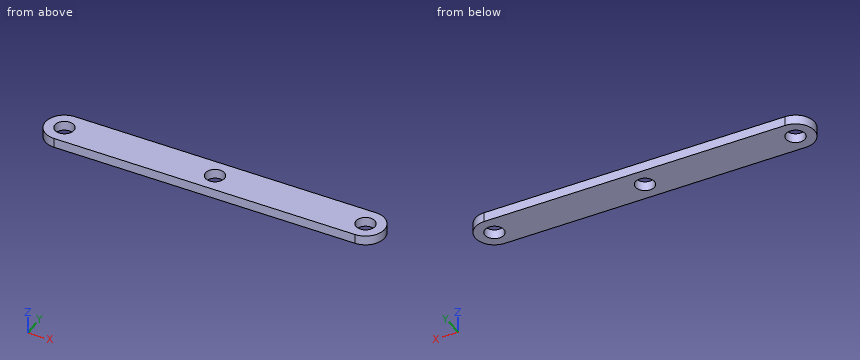
```python
from build123d import *

# Parameters (mm, degrees)
SKETCH1_R           = 3.175
BOSS_EXTRUDE1_DEPTH = 3.175


with BuildPart() as part:
    # Sketch1 → Boss-Extrude1 (new body)
    with BuildSketch(Plane.XY):
        with BuildLine():
            Line((0, 6.35), (101.6, 6.35))
            ThreePointArc((101.6, 6.35), (107.95, 0), (101.6, -6.35))
            Line((101.6, -6.35), (0, -6.35))
            ThreePointArc((0, -6.35), (-6.35, 0), (0, 6.35))
        make_face()
        Circle(SKETCH1_R, mode=Mode.SUBTRACT)
        with Locations((101.6, 0)):
            Circle(SKETCH1_R, mode=Mode.SUBTRACT)
        with Locations((50.8, 0)):
            Circle(SKETCH1_R, mode=Mode.SUBTRACT)
    extrude(amount=BOSS_EXTRUDE1_DEPTH)


solid = part.part
```
Verification items for the finished model (mm, model axes). Give positions to 0.01 mm unless a question says otherwise; leave off trailing zeros. Loops run counter-clockwise (first coordinate to the right, second up) from the corner with the lowest first, then second, coordinate; pieces in that order, holes last. Notation, with made-up numbers: M -9.75,86 L 20.25,86 A13 ccw 20.25,92 Z; hole C -20.75,19 d11. An arc over 180 degrees is marked long. One line per question, with ' | ' between items.
Item 1: Section check A-A, the plane x = 50.8. Record the cut outline in (y, z) (3 decimals), plus the area to 3 significant figures.
Completed:
outline: M -6.35,0 L -3.175,0 L -3.175,3.175 L -6.35,3.175 Z; M 3.175,0 L 6.35,0 L 6.35,3.175 L 3.175,3.175 Z | area: 20.2 mm^2
Item 2: Section check B-B, the plane z = 1.25. Record the cut outline in (x, y) (3 decimals), plus the area to 3 significant figures.
Completed:
outline: M 0,-6.35 L 101.6,-6.35 A6.35 ccw 101.6,6.35 L 0,6.35 A6.35 ccw Z; hole C 0,0 d6.35; hole C 50.8,0 d6.35; hole C 101.6,0 d6.35 | area: 1,320 mm^2
Item 3: Depth check by flat-ended pin: P1, Ø5.5, axis at x = 50.8, y = 0, coming from the -Z side; P2, Ø1, axis at y = -4.5, z = 2, coming from the +X side. Enter the tip coordinate at first touch or a pass-through.
Completed:
P1: passes through | P2: stops at x = 106.53
Item 4: Section check C-C, the plane y = 0. Record the cut outline in (x, z) (3 decimals).
Completed:
outline: M -6.35,0 L -3.175,0 L -3.175,3.175 L -6.35,3.175 Z; M 3.175,0 L 47.625,0 L 47.625,3.175 L 3.175,3.175 Z; M 53.975,0 L 98.425,0 L 98.425,3.175 L 53.975,3.175 Z; M 104.775,0 L 107.95,0 L 107.95,3.175 L 104.775,3.175 Z
Item 5: Thickness scan on line 1 (Y direction, x = 101.6, z = 2.15) (3 decimals); line 2 (X direction, y = 1.75, z = 1.15); line 3 (X direction, y = 2, z = 1). Record the ranges inside material, lowest first. Write a range as [from, to].
Completed:
line 1: y = [-6.35, -3.175], [3.175, 6.35] | line 2: x = [-6.1, -2.65], [2.65, 48.15], [53.45, 98.95], [104.25, 107.7] | line 3: x = [-6.03, -2.47], [2.47, 48.33], [53.27, 99.13], [104.07, 107.63]
